Verification items for this drawing (mm, ordinates from the low corner). Round coordinates to 2 decimals unless told otherwise and drop trailing zeros. Write each loop counter-clockwise with the first axis right and the second up, starting at its lowest first coordinate (ties: lowest second). Pieces come first, ordered by that corner, then holes. Notation, with made-up numbers: (83.5, 70) -> (120.5, 70) arc R22 ccw to (120.5, 82) -> close; hole circle Ø11 at (10, 22.25). An arc over 180 degrees is marked (long way). One line per question, with ' | ' between items.
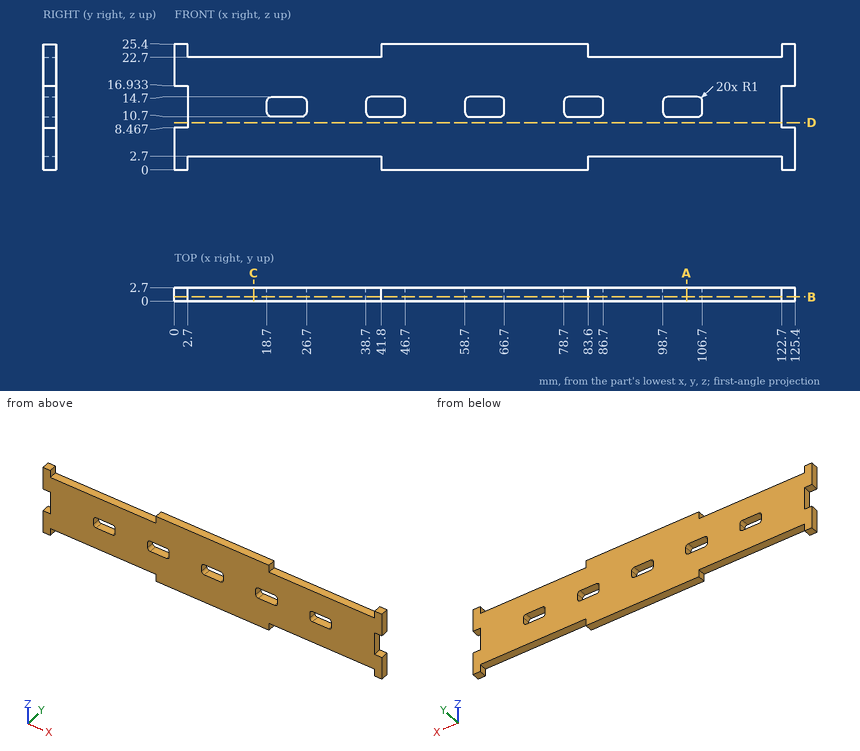
(1) Sectioned sample at B-B on y = 0.85. Count the separate pieces of the cut face and the enclosed holes in it, then the cut area to 3 significant figures.
Resolved:
separate pieces: 1 | enclosed holes: 5 | area: 2,560 mm2
(2) Sectioned sample at D-D on z = 9.5. Record the cut outline in (x, y), then the cut area to 3 significant figures.
Resolved:
outline: (2.7, 0) -> (122.7, 0) -> (122.7, 2.7) -> (2.7, 2.7) -> close | area: 324 mm2
(3) Go/stop test with flat-tipped pins: pin 1 (0.8 mm diameter, centred on x = 123.5, y = 1, fed in from -Z); pin 2 (0.8 mm diameter, centred on x = 25, y = 0.5, fed in from +Z); pin 3 (1.6 mm diameter, centred on y = 1.5, z = 12.5, fed in from -X). Record where each tip stops, or that it passes through.
Resolved:
pin 1: stops at z = 0 | pin 2: stops at z = 22.7 | pin 3: stops at x = 2.7
(4) Sectioned sample at C-C on x = 16. Record the cut outline in (y, z).
Resolved:
outline: (0, 2.7) -> (2.7, 2.7) -> (2.7, 22.7) -> (0, 22.7) -> close
(5) Material ranges on line 1 (X direction, y = 2.2, z = 1); line 2 (X direction, y = 0.4, z = 13.25); line 3 (Z direction, x = 101, y = 1.35), recorded low to high.
Resolved:
line 1: x = 0 to 2.7, 41.8 to 83.6, 122.7 to 125.4 | line 2: x = 2.7 to 18.7, 26.7 to 38.7, 46.7 to 58.7, 66.7 to 78.7, 86.7 to 98.7, 106.7 to 122.7 | line 3: z = 2.7 to 10.7, 14.7 to 22.7
(6) Sectioned sample at A-A on x = 103.5. Record the cut outline in (y, z), then the cut area to 3 significant figures.
Resolved:
outline: (0, 2.7) -> (2.7, 2.7) -> (2.7, 10.7) -> (0, 10.7) -> close; (0, 14.7) -> (2.7, 14.7) -> (2.7, 22.7) -> (0, 22.7) -> close | area: 43.2 mm2
